Geometry: final body of the model. Coordinates: model frame, mm. A direction names the side the tool comes from. Round coordinates to 2 decimals unless told otherwise and drop trailing zeros. Loops run counter-clockwise (first coordinate to the right, second up) from the corner with the lowest first, then second, coordinate; pieces in that order, holes last. Notation, with made-up numbers: (-14.75, 71.5) - (-10.75, 71.5) arc R5 ccw to (-10.75, 76.5) - close; hole circle Ø11 at (15.5, 36.25). An arc over 180 degrees is marked (long way). Use CSV: the item, a comma, the result in double quotes.
from build123d import *

# Parameters (mm, degrees)
SKETCH1_W           = 61
SKETCH1_H           = 61
BOSS_EXTRUDE1_DEPTH = 12.7
SKETCH2_R           = 2
CUT_EXTRUDE1_DEPTH  = 45.964319188
SKETCH3_R           = 3
CUT_EXTRUDE2_DEPTH  = 45.964319188
SKETCH4_W           = 12
SKETCH4_H           = 61
CUT_EXTRUDE3_DEPTH  = 7.7


with BuildPart() as part:
    # Sketch1 → Boss-Extrude1 (new body)
    with BuildSketch(Plane.XY):
        Rectangle(SKETCH1_W, SKETCH1_H)
    extrude(amount=-BOSS_EXTRUDE1_DEPTH)

    # Sketch2 → Cut-Extrude1 (cut, through all)
    with BuildSketch(Plane.XY):
        with Locations((8.838834765, 8.838834765)):
            Circle(SKETCH2_R)
        with Locations((-8.838834765, 8.838834765)):
            Circle(SKETCH2_R)
        with Locations((-8.838834765, -8.838834765)):
            Circle(SKETCH2_R)
        with Locations((8.838834765, -8.838834765)):
            Circle(SKETCH2_R)
    extrude(amount=-CUT_EXTRUDE1_DEPTH, mode=Mode.SUBTRACT)

    # Sketch3 → Cut-Extrude2 (cut, through all)
    with BuildSketch(Plane.XY):
        with Locations((26.5, 20)):
            Circle(SKETCH3_R)
        with Locations((26.5, -20)):
            Circle(SKETCH3_R)
        with Locations((-26.5, 20)):
            Circle(SKETCH3_R)
        with Locations((-26.5, -20)):
            Circle(SKETCH3_R)
    extrude(amount=-CUT_EXTRUDE2_DEPTH, mode=Mode.SUBTRACT)

    # Sketch4 → Cut-Extrude3 (cut)
    with BuildSketch(Plane.XY):
        with Locations((-24.5, 0)):
            Rectangle(SKETCH4_W, SKETCH4_H)
        with Locations((24.5, 0)):
            Rectangle(SKETCH4_W, SKETCH4_H)
    extrude(amount=-CUT_EXTRUDE3_DEPTH, mode=Mode.SUBTRACT)


solid = part.part
Item 1: Section B-B on x = 26.5. Return the cut outline in (y, z), plus the area to 3 significant figures.
Final values:
outline,"(-30.5, -12.7) - (-23, -12.7) - (-23, -7.7) - (-30.5, -7.7) - close; (-17, -12.7) - (17, -12.7) - (17, -7.7) - (-17, -7.7) - close; (23, -12.7) - (30.5, -12.7) - (30.5, -7.7) - (23, -7.7) - close"
area,"245 mm²"
Item 2: Section D-D on z = -11. Give the number of separate pieces and of enclosed holes in the cut face, plus the area to 3 significant figures.
Final values:
separate pieces,"1"
enclosed holes,"8"
area,"3,560 mm²"
Item 3: Material intervals for line 1 (Y direction, x = 26.5, z = -9.8); line 2 (X direction, y = 8.5, z = -4); line 3 (X direction, y = -9.5, z = -6), sorted ascending.
Final values:
line 1,"y = -30.5 to -23, -17 to 17, 23 to 30.5"
line 2,"x = -18.5 to -10.81, -6.87 to 6.87, 10.81 to 18.5"
line 3,"x = -18.5 to -10.73, -6.95 to 6.95, 10.73 to 18.5"
Item 4: Reachability of faces 4 (the cylindrical face through (-28.9, -21.8, -10.2)), 5 (the flat face through (24, 0, -7.7)), 6 (the flat face through (-25, 0, -7.7)) from +Z, -Z, +X, -X, +Y, -Y: full face, straight path, thin tool, end or side. Return the list, or none.
Final values:
face 4,"+Z, -Z"
face 5,"+Z, +X, +Y, -Y"
face 6,"+Z, -X, +Y, -Y"
Item 5: Section C-C on y = 5. Return the cut outline in (x, z), plus the area to 3 significant figures.
Final values:
outline,"(-30.5, -12.7) - (30.5, -12.7) - (30.5, -7.7) - (18.5, -7.7) - (18.5, 0) - (-18.5, 0) - (-18.5, -7.7) - (-30.5, -7.7) - close"
area,"590 mm²"
Item 6: Mould query, pull axis X, two halves, no side actions, for faces 1 (the flat face through (18.5, 0, -4)), 2 (the cylindrical face through (24.1, -21.8, -10.2)), 3 (the flat face through (0, 0, -12.7)). Classes: released by +X, released by -X, zero draft, split by the parting line, or undercut.
Final values:
face 1,"released by +X"
face 2,"undercut"
face 3,"zero draft"
Item 7: Section A-A on y = -20. Return the cut outline in (x, z), plus the area to 3 significant figures.
Final values:
outline,"(-30.5, -12.7) - (-29.5, -12.7) - (-29.5, -7.7) - (-30.5, -7.7) - close; (-23.5, -12.7) - (23.5, -12.7) - (23.5, -7.7) - (18.5, -7.7) - (18.5, 0) - (-18.5, 0) - (-18.5, -7.7) - (-23.5, -7.7) - close; (29.5, -12.7) - (30.5, -12.7) - (30.5, -7.7) - (29.5, -7.7) - close"
area,"530 mm²"
Item 8: Pin query (flat end, axial travel): P1, Ø2.5, axis at x = 8.84, y = 8.84, coming from the +Z side; P2, Ø6, axis at y = -4, z = -2.5, coming from the +X side; P3, Ø2.5, axis at y = 4, z = -3.5, coming from the -X side; P4, Ø8, axis at x = -26.5, y = 20, coming from the +Z side. Return the tip coordinate at first contact, or that it passes through.
Final values:
P1,"passes through"
P2,"stops at x = 18.5"
P3,"stops at x = -18.5"
P4,"stops at z = -7.7"
